The model under review builds one solid part; all positions refer to its coordinate system, in mm. A direction names the side the tool comes from. Coordinates: 2 decimals unless noted, no trailing zeros. Loops run counter-clockwise (first coordinate to the right, second up) from the corner with the lowest first, then second, coordinate; pieces in that order, holes last. Notation, with made-up numbers: M 80,64.25 L 84,64.25 A22 ccw 84,70.25 Z; hole C 25.25,6.25 d2. An arc over 180 degrees is marked long. One line per item, written item: value.
Autodesk Inventor part; units mm, degrees
ref_plane "YZ Plane" through (0, 0, 0) normal (1, 0, 0) x (0, 1, 0)
ref_plane "XZ Plane" through (0, 0, 0) normal (0, 1, 0) x (-1, 0, 0)
ref_plane "XY Plane" through (0, 0, 0) normal (0, 0, 1) x (1, 0, 0)
sketch "Sketch1" plane through (0, 0, 0) normal (0, 0, 1) x (1, 0, 0)
  line L0 (-194.31, -38.1) -> (194.31, -38.1)
  line L1 (194.31, -38.1) -> (194.31, 38.1)
  line L2 (194.31, 38.1) -> (-194.31, 38.1)
  line L3 (-194.31, 38.1) -> (-194.31, -38.1)
  line L4 (-194.31, -38.1) -> (194.31, 38.1) construction
  line L5 (194.31, -38.1) -> (-194.31, 38.1) construction
  line L6 (66, 20) -> (131, 6) construction
  line L7 (131, 20) -> (66, 6) construction
  arc A0 (69.175, 20) -> (66, 16.825) centre (69.175, 16.825) ccw
  arc A1 (66, 9.175) -> (69.175, 6) centre (69.175, 9.175) ccw
  arc A2 (127.825, 6) -> (131, 9.175) centre (127.825, 9.175) ccw
  arc A3 (131, 16.825) -> (127.825, 20) centre (127.825, 16.825) ccw
  line L8 (66, 16.825) -> (66, 9.175)
  line L9 (69.175, 6) -> (127.825, 6)
  line L10 (131, 9.175) -> (131, 16.825)
  line L11 (69.175, 20) -> (127.825, 20)
  line L12 (-131, -6) -> (-66, -20) construction
  line L13 (-66, -6) -> (-131, -20) construction
  arc A4 (-127.825, -6) -> (-131, -9.175) centre (-127.825, -9.175) ccw
  arc A5 (-131, -16.825) -> (-127.825, -20) centre (-127.825, -16.825) ccw
  arc A6 (-69.175, -20) -> (-66, -16.825) centre (-69.175, -16.825) ccw
  arc A7 (-66, -9.175) -> (-69.175, -6) centre (-69.175, -9.175) ccw
  line L14 (-131, -9.175) -> (-131, -16.825)
  line L15 (-127.825, -20) -> (-69.175, -20)
  line L16 (-66, -16.825) -> (-66, -9.175)
  line L17 (-127.825, -6) -> (-69.175, -6)
  arc A8 (-66, 16.825) -> (-69.175, 20) centre (-69.175, 16.825) ccw
  line L18 (-127.825, 20) -> (-69.175, 20)
  line L19 (-127.825, 6) -> (-69.175, 6)
  line L20 (-131, 20) -> (-66, 6) construction
  line L21 (-66, 20) -> (-131, 6) construction
  line L22 (-131, 16.825) -> (-131, 9.175)
  arc A9 (-127.825, 20) -> (-131, 16.825) centre (-127.825, 16.825) ccw
  arc A10 (-131, 9.175) -> (-127.825, 6) centre (-127.825, 9.175) ccw
  line L23 (-66, 9.175) -> (-66, 16.825)
  arc A11 (-69.175, 6) -> (-66, 9.175) centre (-69.175, 9.175) ccw
  arc A12 (131, -9.175) -> (127.825, -6) centre (127.825, -9.175) ccw
  line L24 (69.175, -6) -> (127.825, -6)
  line L25 (69.175, -20) -> (127.825, -20)
  line L26 (66, -6) -> (131, -20) construction
  line L27 (131, -6) -> (66, -20) construction
  line L28 (66, -9.175) -> (66, -16.825)
  arc A13 (69.175, -6) -> (66, -9.175) centre (69.175, -9.175) ccw
  arc A14 (66, -16.825) -> (69.175, -20) centre (69.175, -16.825) ccw
  line L29 (131, -16.825) -> (131, -9.175)
  arc A15 (127.825, -20) -> (131, -16.825) centre (127.825, -16.825) ccw
  point P0 (0, 0)
  point P1 (0, 0)
  point P2 (98.5, 13)
  point P3 (-98.5, -13)
  point P4 (-98.5, 13)
  point P5 (98.5, -13)
  dimension "d0" = 388.62
  dimension "d1" = 76.2
extrude "Extrusion4" add sketch "Sketch1" along normal blind 9.525
properties part number "BK-BKT120-Front" material "Aluminum 6061"
(1) Add section B-B on z = 1.75. State how many separate pieces and enclosed holes the cut face has, then the cut area to 3 significant figures.
Checks:
separate pieces: 1
enclosed holes: 4
area: 26,000 mm^2
(2) Tool access review of faces 1 (the face through (-194.31, 1, 5)), 2 (the face through (98, 6, 5)): name each direction out of +Z, -Z, +X, -X, +Y, -Y from which nothing blocks a thin tool from reaching the whole face with its end or side.
Checks:
face 1: +Z, -Z, -X, +Y, -Y
face 2: +Z, -Z
(3) Add section A-A on x = 91. State the section outline as (y, z) points (3 decimals).
Checks:
outline: M -38.1,0 L -20,0 L -20,9.525 L -38.1,9.525 Z; M -6,0 L 6,0 L 6,9.525 L -6,9.525 Z; M 20,0 L 38.1,0 L 38.1,9.525 L 20,9.525 Z
(4) Insertion check: pin 1 Ø8 at (x, y) = (137, 6.5) entering from -Z. The pin has a flat end and moves straight along its axis. Give the tip position at first contact, or say it passes through.
Checks:
pin 1: z = 0
(5) Draft analysis for pull direction X (two halves, no side actions). For faces 3 (the face through (-3, -38.1, 5)), 4 (the face through (-99, -6, 5)), 5 (the face through (194.31, -1, 5)), state which applies: pulls with the +X half, pulls with the -X half, needs draft (parallel to the pull), parting line crosses it, or undercut.
Checks:
face 3: needs draft
face 4: undercut
face 5: pulls with the +X half
(6) To check wall thickness, follow L1, parallel to X at y = -12, z = 1.5; L2, parallel to X at y = 17.5, z = 0.5; L3, parallel to Y at x = 117.5, z = 5.5. State the ranges of each line that lie inside material, in increasing order. Write a range as [from, to].
Checks:
L1: [-194.31, -131], [-66, 66], [131, 194.31]
L2: [-194.31, -130.93], [-66.07, 66.07], [130.93, 194.31]
L3: [-38.1, -20], [-6, 6], [20, 38.1]
